Part print with two shaded views. Sizes in mm from the minimum x, y, z corner. A direction names the side the tool comes from. Coordinates: 2 decimals unless noted, no trailing zeros. Loops run counter-clockwise (first coordinate to the right, second up) from the corner with the lowest first, then second, coordinate; pieces in that order, holes last. Notation, with made-up numbers: (19.5, 69.5) -> (54.5, 69.5) arc R18 cw to (54.5, 85.5) -> close; hole circle Ø4 at (-13, 23). An arc over 180 degrees is marked (long way). One line per item, written item: value. Start each with the question number.
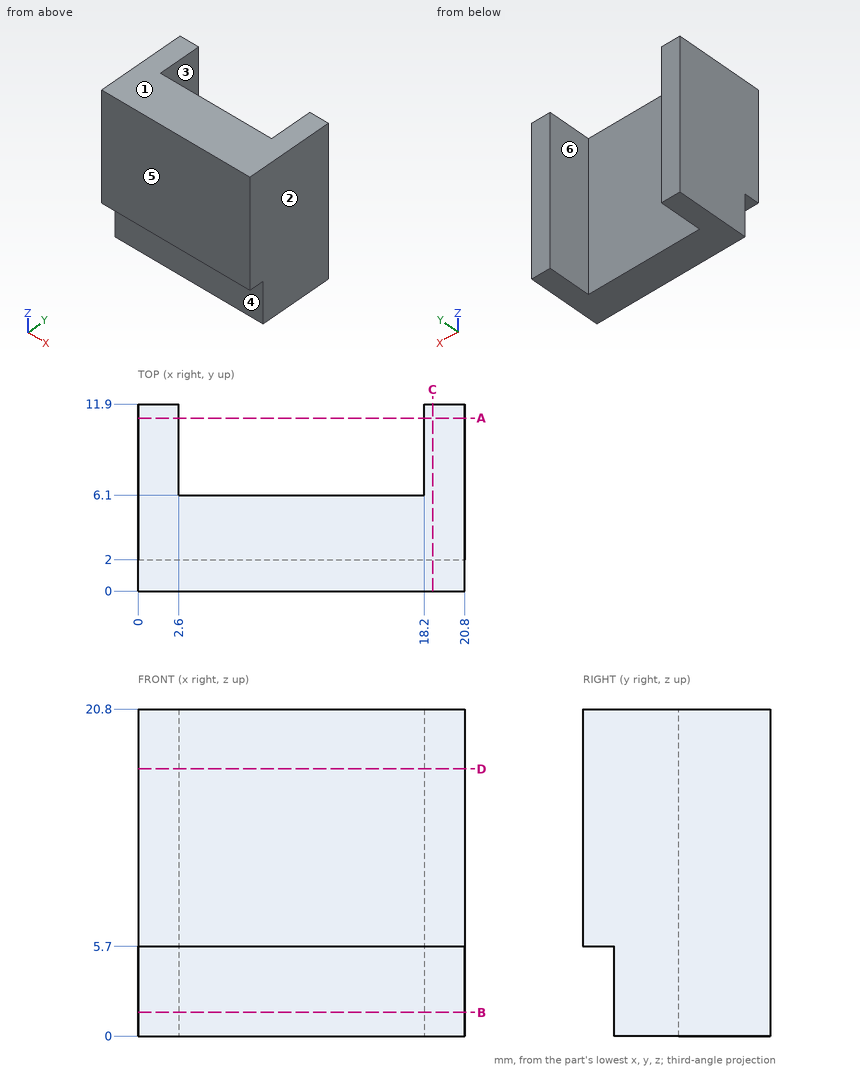
Item 1: Band-saw the part on A-A, the plane y = 11. List the corners of the cut face in (x, z).
Item 2: Probe probe 1 along X at (y, z) = (9, 14); probe 2 along Z at (x, y) = (14, 0.5); probe 3 along Y at (x, z) = (16.25, 14.5). List the from-to ranges inside material, lowest first.
Item 3: Tool access for the marked faces 4, 5 and 6: list every direction of +Z, -Z, +X, -X, +Y, -Y with a clear straight run to the whole face (end or side of a thin tool).
Item 4: Drop flat-ended pins along their axis: pin 1 Ø1.6 at (x, y) = (11, 1) entering from -Z; pin 2 Ø2 at (x, z) = (15.5, 18) entering from +Y. Give the stop position or say it passes through.
Item 5: Band-saw the part on C-C, the plane x = 18.75. List the corners of the cut face in (y, z).
Item 6: Band-saw the part on D-D, the plane z = 17. List the corners of the cut face in (x, y).
Item 7: Two-plate mould, pull along X, no slides. Class the marked faces 1, 2 and 3: +X half, -X half, draft (parallel to the pull), parting line (faces both ways), or undercut.
Item 8: Band-saw the part on B-B, the plane z = 1.5. List the corners of the cut face in (x, y).
Worked out:
1. outline: (0, 0) -> (2.6, 0) -> (2.6, 20.8) -> (0, 20.8) -> close; (18.2, 0) -> (20.8, 0) -> (20.8, 20.8) -> (18.2, 20.8) -> close
2. probe 1: x = 0 to 2.6, 18.2 to 20.8
2. probe 2: z = 5.7 to 20.8
2. probe 3: y = 0 to 6.1
3. face 4: -Z, +X, -X, -Y
3. face 5: +Z, -Z, +X, -X, -Y
3. face 6: +Z, -Z, +Y
4. pin 1: stops at z = 5.7
4. pin 2: stops at y = 6.1
5. outline: (0, 5.7) -> (2, 5.7) -> (2, 0) -> (11.9, 0) -> (11.9, 20.8) -> (0, 20.8) -> close
6. outline: (0, 0) -> (20.8, 0) -> (20.8, 11.9) -> (18.2, 11.9) -> (18.2, 6.1) -> (2.6, 6.1) -> (2.6, 11.9) -> (0, 11.9) -> close
7. face 1: draft
7. face 2: +X half
7. face 3: undercut
8. outline: (0, 2) -> (20.8, 2) -> (20.8, 11.9) -> (18.2, 11.9) -> (18.2, 6.1) -> (2.6, 6.1) -> (2.6, 11.9) -> (0, 11.9) -> close
